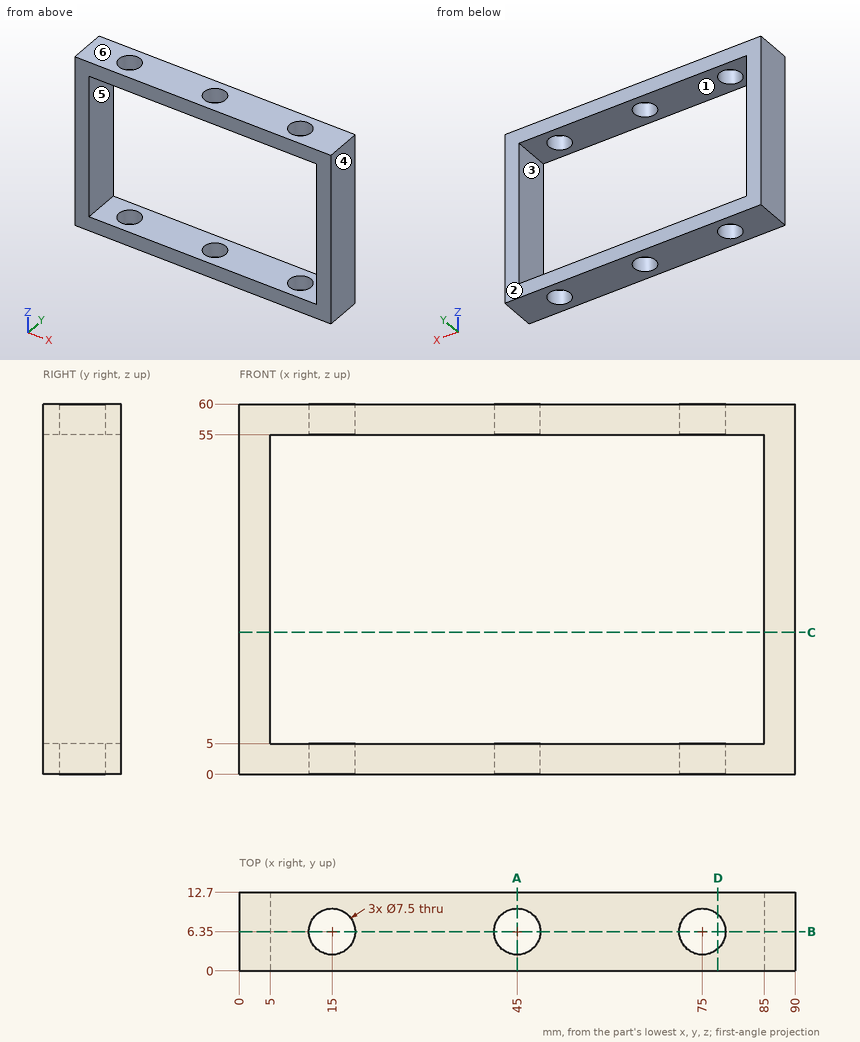
Print and shaded views of the part. All mm, measured from the part's lowest x, y and z. A direction names the side the tool comes from. Coordinates: 2 decimals unless noted, no trailing zeros. Order: outer loops, then holes, each group sorted by start corner. A loop starts at its lowest first (then second) coordinate and runs counter-clockwise, first axis right, second up. Notation, with made-up numbers: (40, 50) - (67, 50) arc R27 cw to (67, 66) - close; hole circle Ø7 at (12.25, -14.75). An arc over 180 degrees is marked (long way). Return JSON: item names as keys, results as strings. Group by question number.
Item 1: Cut at C-C (z = 23). List the corners of the cut face in (x, y), plus the area to 3 significant figures.
Item 2: Cut at A-A (x = 45). List the corners of the cut face in (y, z).
Item 3: Cut at B-B (y = 6.35). State how many separate pieces and enclosed holes the cut face has, plus the area to 4 significant figures.
Item 4: Pull direction X, two halves, no side cores. Call the marked faces 3, 4, 5 and 6: pulls with the +X half, pulls with the -X half, needs draft (parallel to the pull), parting line crosses it, or undercut.
Item 5: Cut at D-D (x = 77.5). List the corners of the cut face in (y, z).
Item 6: Which spindle directions (+Z, -Z, +X, -X, +Y, -Y) get a long thin tool onto all of the face, cutting with end or side? Do the marked faces 1 and 2. Say none if no direction does.
Item 7: Drill centre lines: probe 1 along X at (y, z) = (6.35, 3.65); probe 2 along X at (y, z) = (9.75, 19.5); probe 3 along Z at (x, y) = (30.5, 2.75). Where is each one in solid material? Low to high. Write a range as from..to.
Check values:
{
 "1": {"outline": "(0, 0) - (5, 0) - (5, 12.7) - (0, 12.7) - close; (85, 0) - (90, 0) - (90, 12.7) - (85, 12.7) - close", "area": "127 mm2"},
 "2": {"outline": "(0, 0) - (2.6, 0) - (2.6, 5) - (0, 5) - close; (0, 55) - (2.6, 55) - (2.6, 60) - (0, 60) - close; (10.1, 0) - (12.7, 0) - (12.7, 5) - (10.1, 5) - close; (10.1, 55) - (12.7, 55) - (12.7, 60) - (10.1, 60) - close"},
 "3": {"separate pieces": "6", "enclosed holes": "0", "area": "1,175 mm2"},
 "4": {"face 3": "undercut", "face 4": "pulls with the +X half", "face 5": "undercut", "face 6": "needs draft"},
 "5": {"outline": "(0, 0) - (3.55, 0) - (3.55, 5) - (0, 5) - close; (0, 55) - (3.55, 55) - (3.55, 60) - (0, 60) - close; (9.15, 0) - (12.7, 0) - (12.7, 5) - (9.15, 5) - close; (9.15, 55) - (12.7, 55) - (12.7, 60) - (9.15, 60) - close"},
 "6": {"face 1": "+Y, -Y", "face 2": "+Z, -Z, +X, -X, +Y"},
 "7": {"probe 1": "x = 0..11.25, 18.75..41.25, 48.75..71.25, 78.75..90", "probe 2": "x = 0..5, 85..90", "probe 3": "z = 0..5, 55..60"}
}
